from build123d import *

# Parameters (mm, degrees)
SKETCH1_R           = 4
BOSS_EXTRUDE1_DEPTH = 50
SKETCH2_R           = 5.534283494
SKETCH2_R_2         = 3
CUT_EXTRUDE1_DEPTH  = 15
SKETCH4_R           = 4
SKETCH4_R_2         = 3
CUT_EXTRUDE2_DEPTH  = 15


with BuildPart() as part:
    # Sketch1 → Boss-Extrude1 (new body)
    with BuildSketch(Plane(origin=(0, 0, 0), x_dir=(1, 0, 0), z_dir=(0, 1, 0))):
        with Locations(Location((0, 0, 0), (0, 0, 270))):
            Circle(SKETCH1_R)
    extrude(amount=BOSS_EXTRUDE1_DEPTH)

    # Sketch2 → Cut-Extrude1 (cut)
    with BuildSketch(Plane(origin=(0, 25, 0), x_dir=(1, 0, 0), z_dir=(0, 1, 0))):
        Circle(SKETCH2_R)
        with Locations(Location((0, 0, 0), (0, 0, 270))):
            Circle(SKETCH2_R_2, mode=Mode.SUBTRACT)
    extrude(amount=-CUT_EXTRUDE1_DEPTH, mode=Mode.SUBTRACT)

    # Sketch4 → Cut-Extrude2 (cut)
    with BuildSketch(Plane.XZ.offset(-25)):
        with Locations(Location((0, 0, 0), (0, 0, 90))):
            Circle(SKETCH4_R)
        with Locations(Location((0, 0, 0), (0, 0, 90))):
            Circle(SKETCH4_R_2, mode=Mode.SUBTRACT)
    extrude(amount=-CUT_EXTRUDE2_DEPTH, mode=Mode.SUBTRACT)


solid = part.part
Work out the finished part from the listing and answer in its coordinate system (mm). A direction names the side the tool comes from. Coordinates: 2 decimals unless noted, no trailing zeros. Order: outer loops, then holes, each group sorted by start corner. A loop starts at its lowest first (then second) coordinate and runs counter-clockwise, first axis right, second up. Notation, with made-up numbers: (46, 81.25) - (89, 81.25) arc R12 ccw to (89, 95.25) - close; hole circle Ø3 at (5, 3). An arc over 180 degrees is marked (long way). Put each result on its own line as item: value. Start each with the question number.
1) Find section C-C (y = 25.5). Give the vertices of the cut face in (x, z).
2) For a pull along Y with two mould halves and no side action, classify faces 3 (the flat face through (-3, 40, 1)), 4 (the cylindrical face through (-3.905, 4.93, -0.867)), 5 (the flat face through (1, 10, -3)), 6 (the flat face through (0, 50, 0)) as released by +Y, released by -Y, zero draft, split by the parting line, or undercut.
3) Find section B-B (z = 0). Give the vertices of the cut face in (x, y).
4) Find section A-A (x = 0). Give the vertices of the cut face in (y, z), plus the area to 3 significant figures.
5) Find section D-D (y = 42.5). Give the vertices of the cut face in (x, z), plus the area to 3 significant figures.
6) Flat-ended cylindrical pins translate along their axes: pin 1 (1 mm diameter, centred on x = 2, y = 21.5, fed in from -Z); pin 2 (4 mm diameter, centred on y = 33, z = 2, fed in from +X); pin 3 (4 mm diameter, centred on y = 30.5, z = 1.5, fed in from -X). Find the tip coordinate at first contact, or state that the pin passes through.
7) Find the intervals of material crossed by line 1 (Y direction, x = -2.75, z = 2.5); line 2 (Z direction, x = 0.25, y = 20.5); line 3 (X direction, y = 23, z = 0), in increasing order. Write a range as from..to.
8) For faces 1 (the cylindrical face through (0.9, 25.21, 2.86)), 2 (the flat face through (0, 0, 0)), determine the directions among +Z, -Z, +X, -X, +Y, -Y from which every point of the face is accessible in a straight line to the end or side of a thin tool.
Results list:
1. outline: circle Ø6 at (0, 0)
2. face 3: undercut
2. face 4: zero draft
2. face 5: undercut
2. face 6: released by +Y
3. outline: (-4, 0) - (4, 0) - (4, 10) - (3, 10) - (3, 40) - (4, 40) - (4, 50) - (-4, 50) - (-4, 40) - (-3, 40) - (-3, 10) - (-4, 10) - close
4. outline: (0, -4) - (10, -4) - (10, -3) - (40, -3) - (40, -4) - (50, -4) - (50, 4) - (40, 4) - (40, 3) - (10, 3) - (10, 4) - (0, 4) - close
4. area: 340 mm^2
5. outline: circle Ø8 at (0, 0)
5. area: 50.3 mm^2
6. pin 1: stops at z = -2.6
6. pin 2: stops at x = 3
6. pin 3: stops at x = -3
7. line 1: y = 0..10, 40..50
7. line 2: z = -2.99..2.99
7. line 3: x = -3..3
8. face 1: none
8. face 2: +Z, -Z, +X, -X, -Y
